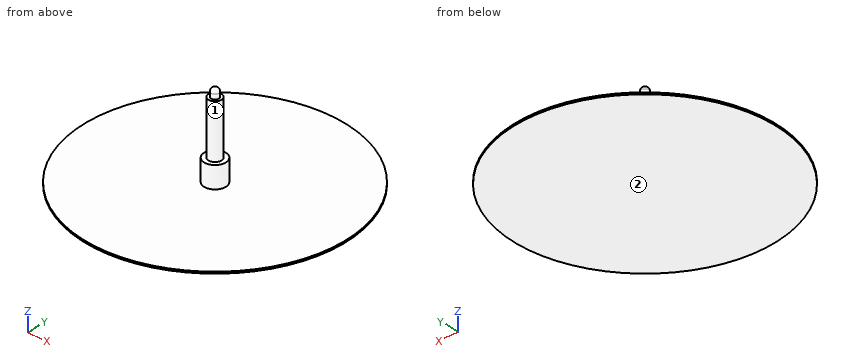
Autodesk Inventor part; units mm, degrees
ref_plane "YZ Plane" through (0, 0, 0) normal (1, 0, 0) x (0, 1, 0)
ref_plane "XZ Plane" through (0, 0, 0) normal (0, 1, 0) x (-1, 0, 0)
ref_plane "XY Plane" through (0, 0, 0) normal (0, 0, 1) x (1, 0, 0)
sketch "Sketch1" plane through (0, 0, 0) normal (0, 0, 1) x (1, 0, 0)
  circle A0 centre (0, 0) radius 300
  dimension "d0" = 600
extrude "Extrusion1" add sketch "Sketch1" along normal blind 4
sketch "Sketch2" plane through (0, 0, 4) normal (0, 0, 1) x (1, 0, 0)
  circle A0 centre (0, 0) radius 300
  circle A1 centre (0, 0) radius 25
  circle A2 centre (0, 0) radius 15
  dimension "d3" = 50
  dimension "d4" = 30
extrude "Extrusion2" add sketch "Sketch2" along normal blind 50 contours A1 | A2
extrude "Extrusion3" add sketch "Sketch2" along normal blind 174 contours A2
sketch "Sketch3" plane through (0, 0, 178) normal (0, 0, 1) x (1, 0, 0)
  circle A0 centre (0, 0) radius 15
  circle A1 centre (0, 0) radius 9
  dimension "d9" = 18
extrude "Extrusion4" add sketch "Sketch3" along normal blind 20 contours A1
fillet "Fillet1" radius 9 1 edges at (-9, 0, 198)
sketch "Sketch4" plane through (0, 0, 4) normal (0, 0, 1) x (1, 0, 0)
  circle A0 centre (0, 0) radius 25
  circle A1 centre (0, 0) radius 300
  line L0 (0, 0) -> (0, 300)
  line L1 (0, 0) -> (0, -300)
  line L2 (0, 0) -> (300, 0)
properties part number "lilin + dudukan + alas"
Verification items for the finished model (mm, model axes). Face numbers are marked on the shaded views. A direction names the side the tool comes from. Round coordinates to 2 decimals unless told otherwise and drop trailing zeros. Write each loop counter-clockwise with the first axis right and the second up, starting at its lowest first coordinate (ties: lowest second). Pieces come first, ordered by that corner, then holes. Notation, with made-up numbers: (-15, -4) - (3, -4) arc R17 cw to (3, 18) - close; hole circle Ø7 at (88, 47.5). An arc over 180 degrees is marked (long way). Answer as a JSON object with one key per item and string values. Group by question number.
Q1. Tool access check on the marked faces 1 and 2. Record the directions out of +Z, -Z, +X, -X, +Y, -Y that give a thin tool (end or side, any length) a straight path to the whole face; none if there is none.
Q2. Section check A-A, the plane y = 0. Enter the section's corners in (x, z), plus the area to 3 significant figures.
Q3. Go/stop test with flat-tipped pins: pin 1 Ø9 at (x, y) = (2, 6.5) entering from +Z; pin 2 Ø8 at (x, z) = (7.5, 94.5) entering from +Y; pin 3 Ø12 at (y, z) = (3.5, 28.5) entering from +X. Record where each tip stops, or that it passes through.
Q4. Section check C-C, the plane z = 169.5. Enter the section's corners in (x, y), plus the area to 3 significant figures.
Q5. Thickness scan on line 1 (Z direction, x = -207, y = 39). Record the ranges inside material, lowest first.
Q6. Section check D-D, the plane y = -152.5. Enter the section's corners in (x, z), plus the area to 3 significant figures.
Found:
{
 "1": {"face 1": "+Z", "face 2": "-Z, +X, -X, +Y, -Y"},
 "2": {"outline": "(-300, 0) - (300, 0) - (300, 4) - (25, 4) - (25, 54) - (15, 54) - (15, 178) - (9, 178) - (9, 189) arc R9 ccw to (-9, 189) - (-9, 178) - (-15, 178) - (-15, 54) - (-25, 54) - (-25, 4) - (-300, 4) - close", "area": "8,950 mm^2"},
 "3": {"pin 1": "stops at z = 197.7", "pin 2": "stops at y = 14.59", "pin 3": "stops at x = 25"},
 "4": {"outline": "circle Ø30 at (0, 0)", "area": "707 mm^2"},
 "5": {"line 1": "z = 0 to 4"},
 "6": {"outline": "(-258.35, 0) - (258.35, 0) - (258.35, 4) - (-258.35, 4) - close", "area": "2,070 mm^2"}
}
